The model under review builds one solid part; all positions refer to its coordinate system, in mm. Face numbers are marked on the shaded views. A direction names the side the tool comes from. Coordinates: 2 decimals unless noted, no trailing zeros. Loops run counter-clockwise (first coordinate to the right, second up) from the corner with the lowest first, then second, coordinate; pieces in that order, holes last. Notation, with made-up numbers: (85, 71.25) -> (99, 71.25) arc R18 ccw to (99, 106.25) -> close; hole circle Ø6 at (66, -37.5). An arc over 180 degrees is marked (long way). One line per question, with ' | ' between items. Start each with the question number.
from build123d import *

# Parameters (mm, degrees)
F0_R     = 1.4
F1_DEPTH = 8
F3_W     = 17.5872370601
F3_H     = 24.5230514556
F4_DEPTH = 0.5
F5_R     = 1.4
F6_DEPTH = 1.5
F7_R     = 1.4
F8_DEPTH = 1.5


with BuildPart() as f1:
    # F0 (on Top) → F1 (new body)
    with BuildSketch(Plane.XY):
        with BuildLine():
            Line((-10.2, 0), (0, 0))
            Line((0, 0), (0, 2.95))
            Line((0, 2.95), (-7, 2.95))
            Line((-7, 2.95), (-7, 15.4))
            Line((-7, 15.4), (2.9, 15.4))
            ThreePointArc((2.9, 15.4), (5.5, 18), (2.9, 20.6))
            Line((2.9, 20.6), (-6.6411852492, 20.6))
            ThreePointArc((-6.6411852492, 20.6), (-7.3482920304, 20.8928932188), (-7.6411852492, 21.6))
            Line((-7.6411852492, 21.6), (-7.6411852492, 22.0574738234))
            ThreePointArc((-7.6411852492, 22.0574738234), (-7.3482920304, 22.7645806046), (-6.6411852492, 23.0574738234))
            Line((-6.6411852492, 23.0574738234), (-3.0835396533, 23.0574738234))
            ThreePointArc((-3.0835396533, 23.0574738234), (-2.4304830107, 23.3001647574), (-2.0944082211, 23.9104397804))
            Line((-2.0944082211, 23.9104397804), (0, 38))
            ThreePointArc((0, 38), (-1.4489432485, 37.5193323495), (-2.4737455949, 36.3878474497))
            Line((-2.4737455949, 36.3878474497), (-10.2, 21.5))
            Line((-10.2, 21.5), (-10.2, 2.95))
            Line((-10.2, 2.95), (-10.2, 0))
        make_face()
        with Locations((0, 18)):
            Circle(F0_R, mode=Mode.SUBTRACT)
    extrude(amount=F1_DEPTH)

    # F3 (on mid) → F4 (join)
    with BuildSketch(Plane.XY.offset(4)):
        with Locations((-4.8047471792, 33.8525986299)):
            Rectangle(F3_W, F3_H)
    extrude(amount=F4_DEPTH)

    # F5 (on face) → F6 (cut)
    with BuildSketch(Plane.XY.offset(8)):
        with BuildLine():
            Line((-7, 20.6665912071), (-7, 15.4))
            Line((-7, 15.4), (2.9, 15.4))
            ThreePointArc((2.9, 15.4), (5.5, 18), (2.9, 20.6))
            Line((2.9, 20.6), (-6.6411852492, 20.6))
            ThreePointArc((-6.6411852492, 20.6), (-6.8236560785, 20.6167887326), (-7, 20.6665912071))
        make_face()
        with Locations((0, 18)):
            Circle(F5_R, mode=Mode.SUBTRACT)
    extrude(amount=-F6_DEPTH, mode=Mode.SUBTRACT)

    # F7 (on face) → F8 (cut)
    with BuildSketch(Plane(origin=(0, 0, 0), x_dir=(1, 0, 0), z_dir=(0, 0, -1))):
        with BuildLine():
            Line((2.9, -15.4), (-7, -15.4))
            Line((-7, -15.4), (-7, -20.6665912071))
            ThreePointArc((-7, -20.6665912071), (-6.8236560785, -20.6167887326), (-6.6411852492, -20.6))
            Line((-6.6411852492, -20.6), (2.9, -20.6))
            ThreePointArc((2.9, -20.6), (5.5, -18), (2.9, -15.4))
        make_face()
        with Locations((0, -18)):
            Circle(F7_R, mode=Mode.SUBTRACT)
    extrude(amount=-F8_DEPTH, mode=Mode.SUBTRACT)


solid = f1.part
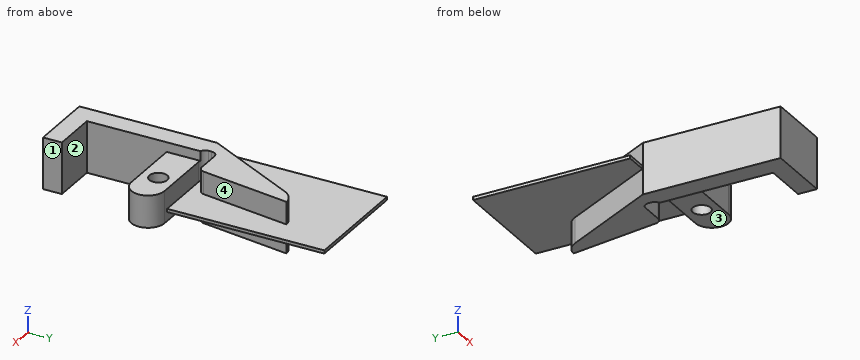
1) Machinability: for the marked faces 1, 2, 3 and 4, which of the approach directions +Z, -Z, +X, -X, +Y, -Y give a long, thin tool a straight path to every point of the face, cutting with its end or side? Answer none if there is none.
2) Consider section A-A, the plane y = 18. Write out the cut boundary in (x, z), plus the area to 3 significant figures.
3) Consider section C-C, the plane x = -6. Write out the cut boundary in (y, z).
4) Consider section D-D, the plane z = 1. Write out the cut boundary in (x, y), plus the area to 3 significant figures.
5) Consider section B-B, the plane z = 5.25. Write out the cut boundary in (x, y).
6) Insertion check: pin 1 Ø5.5 at (x, y) = (-8.5, 32.5) entering from +Z; pin 2 Ø1.8 at (x, z) = (-5.5, 6) entering from -Y; pin 3 Ø6 at (x, y) = (2.5, 18.5) entering from +Z; pin 4 Ø4 at (y, z) = (4.5, 3.5) entering from +X. Each pin has a flat end and moves straight along its axis. Give the tip position at first contact, or say it passes through.
7) Wall thickness on L1, parallel to Y at x = -6.75, z = 2.75; L2, parallel to X at y = 18, z = 2.8; L3, parallel to Z at x = -4, y = 35: over which ranges is each line inside the solid? List them lowest first.
Filled sheet:
1) face 1: +Z, -Z, +X, -Y | face 2: +Z, -Z, +X | face 3: -Z, +X | face 4: +Z, +X
2) outline: (-10.2, 0) -> (-7, 0) -> (-7, 1.5) -> (-1.4, 1.5) -> (-1.4, 6.5) -> (-7, 6.5) -> (-7, 8) -> (-10.2, 8) -> close; (1.4, 1.5) -> (5.5, 1.5) -> (5.5, 6.5) -> (1.4, 6.5) -> close | area: 74.1 mm^2
3) outline: (0, 0) -> (2.95, 0) -> (2.95, 8) -> (0, 8) -> close; (15.4, 1.5) -> (20.6, 1.5) -> (20.6, 6.5) -> (15.4, 6.5) -> close; (21.59, 4) -> (23.06, 4) -> (23.06, 0) -> (29.59, 0) -> (29.59, 4) -> (46.11, 4) -> (46.11, 4.5) -> (29.59, 4.5) -> (29.59, 8) -> (23.06, 8) -> (23.06, 4.5) -> (21.59, 4.5) -> close
4) outline: (-10.2, 0) -> (0, 0) -> (0, 2.95) -> (-7, 2.95) -> (-7, 20.67) arc R1 cw to (-7.64, 21.6) -> (-7.64, 22.06) arc R1 cw to (-6.64, 23.06) -> (-3.08, 23.06) arc R1 ccw to (-2.09, 23.91) -> (0, 38) arc R3 ccw to (-2.47, 36.39) -> (-10.2, 21.5) -> close | area: 158 mm^2
5) outline: (-10.2, 0) -> (0, 0) -> (0, 2.95) -> (-7, 2.95) -> (-7, 15.4) -> (2.9, 15.4) arc R2.6 ccw to (2.9, 20.6) -> (-6.64, 20.6) arc R1 cw to (-7.64, 21.6) -> (-7.64, 22.06) arc R1 cw to (-6.64, 23.06) -> (-3.08, 23.06) arc R1 ccw to (-2.09, 23.91) -> (0, 38) arc R3 ccw to (-2.47, 36.39) -> (-10.2, 21.5) -> close; hole circle Ø2.8 at (0, 18)
6) pin 1: z = 4.5 | pin 2: y = 0 | pin 3: z = 6.5 | pin 4: x = 0
7) L1: 0 to 2.95, 15.4 to 20.61, 23.05 to 28.15 | L2: -10.2 to -1.4, 1.4 to 5.5 | L3: 4 to 4.5
